Can you work these out from the model? Positions are in its coordinate system, mm. Face numbers are marked on the shaded views. A direction names the side the tool comes from. Round coordinates to 2 decimals unless told otherwise and drop trailing zeros. Use CSV: the item, a comma, the result in double quotes.
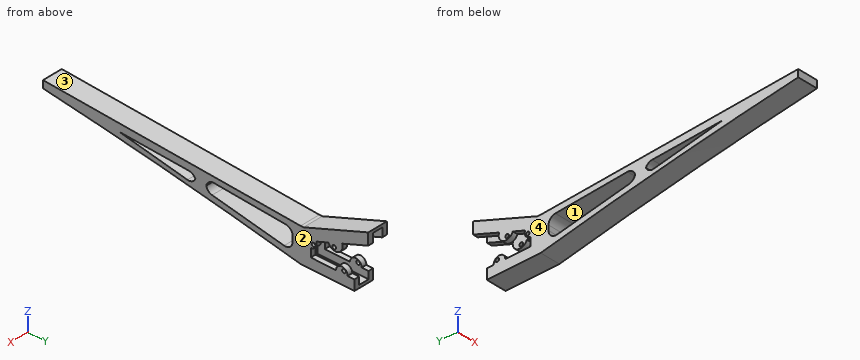
```python
from build123d import *

# Parameters (mm, degrees)
BOSS_EXTRUDE1_DEPTH  = 35
SKETCH6_W            = 14
SKETCH6_H            = 23
BOSS_EXTRUDE6_DEPTH  = 2
BOSS_EXTRUDE8_DEPTH  = 3.5
BOSS_EXTRUDE9_START  = -14
SKETCH14_R           = 1.25
BOSS_EXTRUDE9_DEPTH  = 14
BOSS_EXTRUDE10_DEPTH = 3.5
BOSS_EXTRUDE11_START = -14
SKETCH16_R           = 1.25
BOSS_EXTRUDE11_DEPTH = 14
BOSS_EXTRUDE12_START = -14
SKETCH18_R           = 1.25
BOSS_EXTRUDE12_DEPTH = 14
SKETCH19_W           = 7
SKETCH19_H           = 19
CUT_EXTRUDE5_DEPTH   = 57.095900028
SKETCH20_W           = 7
SKETCH20_H           = 47.4605099
CUT_EXTRUDE6_DEPTH   = 10
BOSS_EXTRUDE13_DEPTH = 14
FILLET1_R            = 5


with BuildPart() as part:
    # Sketch1 → Boss-Extrude1 (new body)
    with BuildSketch(Plane(origin=(0, 0, 0), x_dir=(1, 0, 0), z_dir=(0, 1, 0))):
        Polygon((7, 0), (10.5, 0), (10.5, 7), (-3.5, 7), (-3.5, 0), (0, 0), (0, 5), (7, 5), align=None)
    extrude(amount=BOSS_EXTRUDE1_DEPTH)

    # Sketch6 → Boss-Extrude6 (add)
    with BuildSketch(Plane.XZ):
        with Locations((3.5, 4.5)):
            Rectangle(SKETCH6_W, SKETCH6_H)
    extrude(amount=BOSS_EXTRUDE6_DEPTH)

    # Sweep1: sweep along a path in Sketch8
    with BuildLine(Plane(origin=(10.5, 0, 0), x_dir=(0, 0, -1), z_dir=(1, 0, 0))) as sweep1_path:
        Line((-32.5, 44.5), (-16, 0))
    # Sketch7 → Sweep1 (sweep)
    with BuildSketch(Plane(origin=(0, 0, 0), x_dir=(1, 0, 0), z_dir=(0, 1, 0))):
        Polygon((-3.5, -16), (10.5, -16), (10.5, -8), (7, -8), (7, -14), (0, -14), (0, -8), (-3.5, -8), align=None)
    sweep(path=sweep1_path.line)

    # Sketch13 → Boss-Extrude8 (add)
    with BuildSketch(Plane(origin=(10.5, 0, 0), x_dir=(0, 0, -1), z_dir=(1, 0, 0))):
        Polygon((-8, 0), (0, 0), (0, 5), (-9.853932584, 5), align=None)
    extrude(amount=-BOSS_EXTRUDE8_DEPTH)

    # Sketch14 → Boss-Extrude9 (add)
    with BuildSketch(Plane(origin=(10.5, 0, 0), x_dir=(0, 0, -1), z_dir=(1, 0, 0)).offset(BOSS_EXTRUDE9_START)):
        with BuildLine():
            Line((-9.853932584, 5), (-11.243474968, 8.747553701))
            ThreePointArc((-11.243474968, 8.747553701), (-7.571262705, 8.280915268), (-5.85706046, 5))
            Line((-5.85706046, 5), (-9.853932584, 5))
        make_face()
        with Locations((-8.532023173, 6.9)):
            Circle(SKETCH14_R, mode=Mode.SUBTRACT)
    extrude(amount=BOSS_EXTRUDE9_DEPTH)

    # Sketch15 → Boss-Extrude10 (add)
    with BuildSketch(Plane.ZY.offset(3.5)):
        Polygon((0, 0), (8, 0), (9.853932584, 5), (0, 5), align=None)
    extrude(amount=-BOSS_EXTRUDE10_DEPTH)

    # Sketch16 → Boss-Extrude11 (add)
    with BuildSketch(Plane(origin=(10.5, 0, 0), x_dir=(0, 0, -1), z_dir=(1, 0, 0)).offset(BOSS_EXTRUDE11_START)):
        with BuildLine():
            ThreePointArc((0, 30.317524518), (-4, 26.317524518), (0, 22.317524518))
            Line((0, 22.317524518), (0, 26.317524518))
            Line((0, 26.317524518), (0, 30.317524518))
        make_face()
        with Locations((-1.9, 27.817524518)):
            Circle(SKETCH16_R, mode=Mode.SUBTRACT)
    extrude(amount=BOSS_EXTRUDE11_DEPTH)

    # Sketch18 → Boss-Extrude12 (add)
    with BuildSketch(Plane(origin=(10.5, 0, 0), x_dir=(0, 0, -1), z_dir=(1, 0, 0)).offset(BOSS_EXTRUDE12_START)):
        with BuildLine():
            Line((-17.848966579, 26.562364409), (-14.372392047, 17.186148247))
            ThreePointArc((-14.372392047, 17.186148247), (-11.422571232, 23.612543594), (-17.848966579, 26.562364409))
        make_face()
        with Locations((-13.310679313, 21.074256328)):
            Circle(SKETCH18_R, mode=Mode.SUBTRACT)
    extrude(amount=BOSS_EXTRUDE12_DEPTH)

    # Sketch19 → Cut-Extrude5 (cut, through all)
    with BuildSketch(Plane(origin=(0, 0, 0), x_dir=(1, 0, 0), z_dir=(0, 1, 0))):
        with Locations((3.5, -4.5)):
            Rectangle(SKETCH19_W, SKETCH19_H)
    extrude(amount=CUT_EXTRUDE5_DEPTH, mode=Mode.SUBTRACT)

    # Sketch20 → Cut-Extrude6 (cut)
    with BuildSketch(Plane(origin=(0, -4.563596004, 12.307880133), x_dir=(-1, 0, 0), z_dir=(0, 0.3476574532100169, -0.9376216162330756))):
        with Locations((-3.5, 28.597459295)):
            Rectangle(SKETCH20_W, SKETCH20_H)
    extrude(amount=CUT_EXTRUDE6_DEPTH, mode=Mode.SUBTRACT)

    # Sketch9 → Boss-Extrude13 (add)
    with BuildSketch(Plane(origin=(10.5, 0, 0), x_dir=(0, 0, -1), z_dir=(1, 0, 0))):
        with BuildLine():
            Line((-16, -2), (-26, -179))
            Line((-26, -179), (-21, -179))
            add(Edge.make_bspline(
                [(7, -2), (-9.660155009, -89.83535791), (-21, -179)],
                knots=[0, 0, 0, 0.89649965, 0.89649965, 0.89649965], degree=2))
            Line((7, -2), (-16, -2))
        make_face()
        Polygon((-5.08325747, -7.433503799), (-12.08325747, -7.433503799), (-16, -66.930407946), (-8.514117769, -66.930407946), (1.91674253, -7.433503799), align=None, mode=Mode.SUBTRACT)
        Polygon((-12.215264572, -73.873780488), (-15.215264572, -73.873780488), (-17.9028805, -126.858413083), (-8.514117769, -73.873780488), align=None, mode=Mode.SUBTRACT)
    extrude(amount=-BOSS_EXTRUDE13_DEPTH)

    # Fillet1
    # the kernel refuses this fillet: 5 mm, written as the material it adds along each edge
    with BuildSketch(Plane(origin=(10.5, -73.873780488, 8.514117769), x_dir=(0, 0, 1), z_dir=(-1, 0, 0))) as fillet1_piece_1:
        with BuildLine():
            CenterArc((FILLET1_R * 1.19277604339, -FILLET1_R), FILLET1_R, 90, 100.048385075)
            Line((FILLET1_R * 0.208115283733, -FILLET1_R * 1.17447976499), (0, 0))
            Line((0, 0), (FILLET1_R * 1.19277604339, 0))
        make_face()
    extrude(amount=14)
    with BuildSketch(Plane(origin=(10.5, -73.873780488, 15.215264572), x_dir=(0, 0, -1), z_dir=(-1, 0, 0))) as fillet1_piece_2:
        with BuildLine():
            CenterArc((FILLET1_R * 0.950561215954, FILLET1_R), FILLET1_R, 182.903807688, 87.096192312)
            Line((-FILLET1_R * 0.048154776785, FILLET1_R * 0.949340688451), (0, 0))
            Line((0, 0), (FILLET1_R * 0.950561215954, 0))
        make_face()
    extrude(amount=14)
    with BuildSketch(Plane(origin=(10.5, -66.930407946, 16), x_dir=(0, 0, -1), z_dir=(-1, 0, 0))) as fillet1_piece_3:
        with BuildLine():
            CenterArc((FILLET1_R * 1.06799555055, -FILLET1_R), FILLET1_R, 90, 93.766405645)
            Line((FILLET1_R * 0.0701553952566, -FILLET1_R * 1.06568884601), (0, 0))
            Line((0, 0), (FILLET1_R * 1.06799555055, 0))
        make_face()
    extrude(amount=14)
    with BuildSketch(Plane(origin=(10.5, -66.930407946, 8.514117769), x_dir=(0, 0.9849772856062504, -0.17268395073006315), z_dir=(-1, 0, 0))) as fillet1_piece_4:
        with BuildLine():
            CenterArc((FILLET1_R * 0.839934139964, -FILLET1_R), FILLET1_R, 90, 80.056093562)
            Line((-FILLET1_R * 0.145043145642, -FILLET1_R * 0.82731604927), (0, 0))
            Line((0, 0), (FILLET1_R * 0.839934139964, 0))
        make_face()
    extrude(amount=14)
    with BuildSketch(Plane(origin=(10.5, -7.433503799, 12.08325747), x_dir=(0, 0, -1), z_dir=(-1, 0, 0))) as fillet1_piece_5:
        with BuildLine():
            CenterArc((FILLET1_R * 0.936333488925, FILLET1_R), FILLET1_R, 183.766405645, 86.233594355)
            Line((-FILLET1_R * 0.0615066663657, FILLET1_R * 0.934311153992), (0, 0))
            Line((0, 0), (FILLET1_R * 0.936333488925, 0))
        make_face()
    extrude(amount=14)
    with BuildSketch(Plane(origin=(10.5, -7.433503799, -1.91674253), x_dir=(0, 0, 1), z_dir=(-1, 0, 0))) as fillet1_piece_6:
        with BuildLine():
            CenterArc((FILLET1_R * 1.19056953685, -FILLET1_R), FILLET1_R, 90, 99.943906438)
            Line((FILLET1_R * 0.205592251242, -FILLET1_R * 1.17268395073), (0, 0))
            Line((0, 0), (FILLET1_R * 1.19056953685, 0))
        make_face()
    extrude(amount=14)


solid = part.part
```
Q1. If we mould it in two halves opening along Y, with no side actions, what happens to the marked faces 3 and 4? For each: released by +Y, released by -Y, zero draft, split by the parting line, or undercut.
Resolved:
face 3,"undercut"
face 4,"zero draft"
Q2. On a 3-axis mill with a long thin cutter (end or side, diameter ignored), from which of +Z, -Z, +X, -X, +Y, -Y can I reach the whole of each face in a straight line? I mean the marked faces 1 and 2. Say none if no direction works.
Resolved:
face 1,"+X, -X"
face 2,"+Z, -Z, +X, +Y, -Y"
Q3. Please list where these lines run through material, in increasing order: probe 1 along Z at (x, y) = (7.85, 6.9); probe 2 along Z at (x, y) = (8, -105.5); probe 3 along Z at (x, y) = (9.25, -23.5).
Resolved:
probe 1,"z = -7 to 0, 6.34 to 7.28, 9.78 to 18.56"
probe 2,"z = 10.71 to 14.12, 16.82 to 21.85"
probe 3,"z = -3.01 to 0.9, 13.14 to 17.21"
Q4. Suppose I cut it at A-A (x = 4.75). Count the separate pieces of the cut face and the enclosed holes in it, and give its area (3 significant figures).
Resolved:
separate pieces,"1"
enclosed holes,"2"
area,"1,740 mm^2"
Q5. Will these pins go through, and if not, where does the flat tip stop? P1, Ø0.6, axis at x = 0.5, y = -0.5, coming from the +Z side; P2, Ø5, axis at x = 7, y = -17.5, coming from the +Z side; P3, Ø1.8, axis at x = -1.5, y = 17.5, coming from the +Z side.
Resolved:
P1,"stops at z = 16"
P2,"stops at z = 17.02"
P3,"stops at z = 22.82"
